Verification items for the finished model (mm, model axes). A direction names the side the tool comes from. Coordinates: 2 decimals unless noted, no trailing zeros. Answer in a Markdown table with one row per item.
```python
from build123d import *

# Parameters (mm, degrees)
SKETCH1_W                     = 6
SKETCH1_H                     = 35
BOSS_EXTRUDE1_DEPTH           = 1.7
BOSS_EXTRUDE1_TAPER           = 5
BOSS_EXTRUDE1_OTHER_WAY_DEPTH = 1.7
BOSS_EXTRUDE1_OTHER_WAY_TAPER = 5
SKETCH2_W                     = 1.5
SKETCH2_H                     = 0.41
CUT_EXTRUDE1_DEPTH            = 1.7


with BuildPart() as part:
    # Sketch1 → Boss-Extrude1 (new body)
    with BuildSketch(Plane(origin=(0, 0, 0), x_dir=(1, 0, 0), z_dir=(0, 1, 0))):
        with Locations((3, 17.5)):
            Rectangle(SKETCH1_W, SKETCH1_H)
    extrude(amount=BOSS_EXTRUDE1_DEPTH, taper=BOSS_EXTRUDE1_TAPER)

    # Sketch1 → Boss-Extrude1 other way (add)
    with BuildSketch(Plane(origin=(0, 0, 0), x_dir=(1, 0, 0), z_dir=(0, 1, 0))):
        with Locations((3, 17.5)):
            Rectangle(SKETCH1_W, SKETCH1_H)
    extrude(amount=-BOSS_EXTRUDE1_OTHER_WAY_DEPTH, taper=BOSS_EXTRUDE1_OTHER_WAY_TAPER)

    # Sketch2 → Cut-Extrude1 (cut)
    with BuildSketch(Plane(origin=(5.954423259, -0.520944533, 0), x_dir=(0, 0, -1), z_dir=(0.996194698, -0.087155743, 0))):
        with Locations((1.25, 0.317934456)):
            Rectangle(SKETCH2_W, SKETCH2_H)
        with Locations((3.75, 0.317934456)):
            Rectangle(SKETCH2_W, SKETCH2_H)
        with Locations((6.25, 0.317934456)):
            Rectangle(SKETCH2_W, SKETCH2_H)
        with Locations((8.75, 0.317934456)):
            Rectangle(SKETCH2_W, SKETCH2_H)
        with Locations((11.25, 0.317934456)):
            Rectangle(SKETCH2_W, SKETCH2_H)
        with Locations((13.75, 0.317934456)):
            Rectangle(SKETCH2_W, SKETCH2_H)
        with Locations((16.25, 0.317934456)):
            Rectangle(SKETCH2_W, SKETCH2_H)
        with Locations((18.75, 0.317934456)):
            Rectangle(SKETCH2_W, SKETCH2_H)
        with Locations((21.25, 0.317934456)):
            Rectangle(SKETCH2_W, SKETCH2_H)
        with Locations((23.75, 0.317934456)):
            Rectangle(SKETCH2_W, SKETCH2_H)
        with Locations((26.25, 0.317934456)):
            Rectangle(SKETCH2_W, SKETCH2_H)
        with Locations((28.75, 0.317934456)):
            Rectangle(SKETCH2_W, SKETCH2_H)
        with Locations((31.25, 0.317934456)):
            Rectangle(SKETCH2_W, SKETCH2_H)
        with Locations((33.75, 0.317934456)):
            Rectangle(SKETCH2_W, SKETCH2_H)
    cut_extrude1 = extrude(amount=-CUT_EXTRUDE1_DEPTH, mode=Mode.SUBTRACT)

    # Mirror1: Cut-Extrude1 across plane
    add(cut_extrude1.mirror(Plane(origin=(3, 0, 0), x_dir=(0, 0, 1), z_dir=(1, 0, 0))), mode=Mode.SUBTRACT)


solid = part.part
```
1. Section check A-A, the plane x = 1.25. State how many separate pieces and enclosed holes the cut face has, plus the area to 3 significant figures.
Geometry says:
| item | result |
|---|---|
| separate pieces | 1 |
| enclosed holes | 14 |
| area | 110 mm^2 |
2. Tool access check on faces 5 (the flat face through (5.165, 0.073, -11.24)), 6 (the flat face through (0.871, -0.335, -21.24)), 7 (the flat face through (5.129, -0.335, -18.74)), 8 (the flat face through (3, 1.7, -17)). Record the directions out of +Z, -Z, +X, -X, +Y, -Y that give a thin tool (end or side, any length) a straight path to the whole face; none if there is none.
Geometry says:
| item | result |
|---|---|
| face 5 | none |
| face 6 | -X |
| face 7 | +X |
| face 8 | +Z, -Z, +X, -X, +Y |
3. Thickness scan on line 1 (Y direction, x = 5.75, z = -29); line 2 (Y direction, x = 5, z = -13.5); line 3 (Z direction, x = 5.25, y = -1.3). Record the ranges inside material, lowest first. Write a range as from..to.
Geometry says:
| item | result |
|---|---|
| line 1 | -1.7..-0.39, 0.02..1.7 |
| line 2 | -1.7..-0.32, 0.09..1.7 |
| line 3 | -34.89..-0.11 |
4. Mould release check, pull along X, two halves, no side actions. Record for faces 1 (the flat face through (0.835, 0.073, -8.74)), 2 (the flat face through (0.835, 0.073, -1.24)), 3 (the flat face through (0.871, -0.335, -28.74)), 4 (the flat face through (5.129, -0.335, -26.24)): released by +X, released by -X, zero draft, split by the parting line, or undercut.
Geometry says:
| item | result |
|---|---|
| face 1 | undercut |
| face 2 | undercut |
| face 3 | released by -X |
| face 4 | released by +X |
